Autodesk Inventor part; units mm, degrees
ref_plane "YZ Plane" through (0, 0, 0) normal (1, 0, 0) x (0, 1, 0)
ref_plane "XZ Plane" through (0, 0, 0) normal (0, 1, 0) x (-1, 0, 0)
ref_plane "XY Plane" through (0, 0, 0) normal (0, 0, 1) x (1, 0, 0)
sketch "Esquisse1" plane through (0, 0, 0) normal (0, 0, 1) x (1, 0, 0)
  line L0 (-583.7545, 1063.2671) -> (466.2455, 1063.2671)
  line L1 (466.2455, 1063.2671) -> (466.2455, -1086.7329)
  line L2 (466.2455, -1086.7329) -> (-583.7545, -1086.7329)
  line L3 (-583.7545, -1086.7329) -> (-583.7545, 1063.2671)
  point P0 (0, 0)
  dimension "d0" = 1050
  dimension "d1" = 2150
extrude "Extrusion1" add sketch "Esquisse1" along normal blind 1000
sketch "Esquisse2" plane through (-583.7545, 1063.2671, 0) normal (0, 1, 0) x (1, 0, 0)
  line L0 (0, 0) -> (0, -1000)
  line L1 (1050, -1000) -> (0, -1000)
  line L2 (0, -200) -> (1010, -200)
  line L3 (1010, -200) -> (1010, -1000)
  line L4 (1010, -1000) -> (0, -1000)
  line L5 (0, -1000) -> (0, -200)
  line L6 (1050, 0) -> (1050, -1000)
  point P0 (583.7545, 0)
  dimension "d4" = 200
  dimension "d5" = 40
extrude "Extrusion2" cut sketch "Esquisse2" against normal through all
sketch "Esquisse3" plane through (-583.7545, 1063.2671, 200) normal (0, 0, 1) x (1, 0, 0)
  line L0 (1050, -2150) -> (0, -2150)
  line L1 (50, -50) -> (1010.0305, -50)
  line L2 (1010.0305, -50) -> (1010.0305, -2150)
  line L3 (1010.0305, -2150) -> (50, -2150)
  line L4 (50, -2150) -> (50, -50)
  line L5 (0, -2150) -> (0, 0)
  point P0 (583.7545, -1063.2671)
  dimension "d8" = 50
  dimension "d9" = 50
extrude "Extrusion3" cut sketch "Esquisse3" against normal through all
properties part number "Porte Simple" material "Bois (Chêne)"
Source: CAD feature listing. Evaluate the final solid. Frame: model axes, mm. A direction names the side the tool comes from. Give positions to 0.01 mm unless a question says otherwise; leave off trailing zeros. Order: outer loops, then holes, each group sorted by start corner. A loop starts at its lowest first (then second) coordinate and runs counter-clockwise, first axis right, second up. Notation, with made-up numbers: (-3.5, 42.5) -> (47.5, 42.5) arc R28 cw to (47.5, 70.5) -> close; hole circle Ø11 at (64.5, 4). An arc over 180 degrees is marked (long way). Use a Markdown table: item, result.
Q1. Access query for faces 4 (the face through (-533.754, -51, 101)), 5 (the face through (-567, 471, 200)), 6 (the face through (446, 3, 1000)). Directions: +Z, -Z, +X, -X, +Y, -Y. A direction counts if a zero-diameter tool reaches every point of the face in a straight line with its end or side. Return the directions, or none.
A:
| item | result |
|---|---|
| face 4 | +Z, -Z, -Y |
| face 5 | +Z, -X, +Y, -Y |
| face 6 | +Z, +X, -X, +Y, -Y |
Q2. Section C-C (x = -334). Return the cut outline in (y, z), and give its area (3 significant figures).
A:
| item | result |
|---|---|
| outline | (1013.27, 0) -> (1063.27, 0) -> (1063.27, 200) -> (1013.27, 200) -> close |
| area | 10,000 mm^2 |
Q3. Material intervals for line 1 (X direction, y = -483.5, z = 152); line 2 (X direction, y = 915, z = 306.5), sorted ascending. Write a range as [from, to].
A:
| item | result |
|---|---|
| line 1 | [-583.75, -533.75], [426.28, 466.25] |
| line 2 | [426.25, 466.25] |
Q4. Pull-direction query (X, two-part tool) for faces 1 (the face through (466.246, 3, 493)), 2 (the face through (-60, 1013.267, 101)), 3 (the face through (17, 1063.267, 164)); classes: +X half, -X half, draft (parallel to the pull), parting line (faces both ways), or undercut.
A:
| item | result |
|---|---|
| face 1 | +X half |
| face 2 | undercut |
| face 3 | draft |
Q5. First-contact query: P1, Ø4, axis at y = 104, z = 578, coming from the -X side. Flat tip, straight axial feed; report the tip coordinate or a pass-through.
A:
| item | result |
|---|---|
| P1 | x = 426.25 |
Q6. Section D-D (z = 277). Return the cut outline in (x, y), and give its area (3 significant figures).
A:
| item | result |
|---|---|
| outline | (426.25, -1086.73) -> (466.25, -1086.73) -> (466.25, 1063.27) -> (426.25, 1063.27) -> close |
| area | 86,000 mm^2 |
Q7. Section B-B (z = 109). Return the cut outline in (x, y).
A:
| item | result |
|---|---|
| outline | (-583.75, -1086.73) -> (-533.75, -1086.73) -> (-533.75, 1013.27) -> (426.28, 1013.27) -> (426.28, -1086.73) -> (466.25, -1086.73) -> (466.25, 1063.27) -> (-583.75, 1063.27) -> close |
